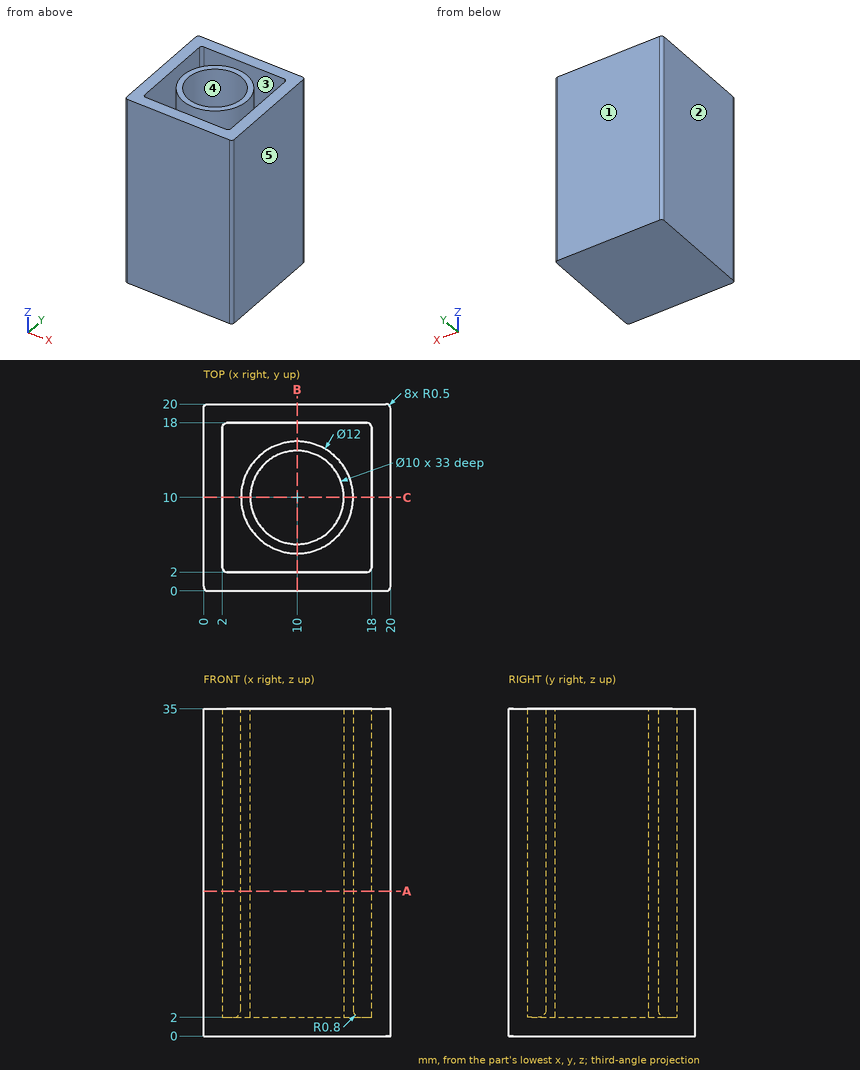
Can you work these out from the drawing? Everything is in mm from the part's minimum corner. A direction names the side the tool comes from. Give positions to 0.01 mm unless a question says otherwise; leave off trailing zeros. Write each loop counter-clockwise with the first axis right and the second up, starting at its lowest first coordinate (ties: lowest second). Pieces come first, ordered by that corner, then holes. Notation, with made-up numbers: (15.25, 61.5) -> (57.25, 61.5) arc R31 cw to (57.25, 95.5) -> close; hole circle Ø8 at (-39.5, -25). An arc over 180 degrees is marked (long way). Write each question's results on one line, items separated by ' | '. Start each with the question number.
Q1. I'm going to push a flat-ended pin straight in: pin 1 Ø5 at (x, y) = (10, 10) entering from +Z. Where does the tip first touch, or does it pass through?
Q2. Suppose I cut it at B-B, the plane x = 10. List the corners of the cut face in (y, z) for me.
Q3. Which directions (+Z, -Z, +X, -X, +Y, -Y) give clear straight access to the entire face, cutting with the end or side of a thin tool? Please do the marked faces 4 and 5.
Q4. Suppose I cut it at A-A, the plane z = 15.5. List the corners of the cut face in (x, y) for me, and give its area (3 significant figures).
Q5. We'd pull the mould along X, two halves only. Please class the marked faces 1, 2 and 3: +X half, -X half, draft (parallel to the pull), parting line (faces both ways), or undercut.
Q6. I need wall thicknesses on probe 1 along Y at (x, z) = (10, 16); probe 2 along Y at (x, z) = (3.25, 3); probe 3 along X at (y, z) = (13.5, 9). Which ranges of each line are inside material? Lowest first, please.
Outcome:
1) pin 1: z = 2
2) outline: (0, 0) -> (20, 0) -> (20, 35) -> (18, 35) -> (18, 2) -> (16.8, 2) arc R0.8 cw to (16, 2.8) -> (16, 35) -> (15, 35) -> (15, 2) -> (5, 2) -> (5, 35) -> (4, 35) -> (4, 2.8) arc R0.8 cw to (3.2, 2) -> (2, 2) -> (2, 35) -> (0, 35) -> close
3) face 4: +Z | face 5: +Z, -Z, +X, +Y, -Y
4) outline: (0, 0.5) arc R0.5 ccw to (0.5, 0) -> (19.5, 0) arc R0.5 ccw to (20, 0.5) -> (20, 19.5) arc R0.5 ccw to (19.5, 20) -> (0.5, 20) arc R0.5 ccw to (0, 19.5) -> close; circle Ø12 at (10, 10); hole (2, 2.5) arc R0.5 ccw to (2.5, 2) -> (17.5, 2) arc R0.5 ccw to (18, 2.5) -> (18, 17.5) arc R0.5 ccw to (17.5, 18) -> (2.5, 18) arc R0.5 ccw to (2, 17.5) -> close; hole circle Ø10 at (10, 10) | area: 179 mm2
5) face 1: draft | face 2: -X half | face 3: undercut
6) probe 1: 0 to 2, 4 to 5, 15 to 16, 18 to 20 | probe 2: 0 to 2, 18 to 20 | probe 3: 0 to 2, 5.13 to 6.43, 13.57 to 14.87, 18 to 20
